```python
from build123d import *

# Parameters (mm, degrees)
SKETCH3_W            = 19.970710678
SKETCH3_H            = 7.220710678
BOSS_EXTRUDE2_DEPTH  = 10
SKETCH4_W            = 54.526496071
SKETCH4_H            = 10
BOSS_EXTRUDE3_DEPTH  = 10
SKETCH5_W            = 7.25
SKETCH5_H            = 10.1
BOSS_EXTRUDE4_DEPTH  = 20
SKETCH6_W            = 54.470710678
SKETCH6_H            = 10
BOSS_EXTRUDE5_DEPTH  = 10
SKETCH7_R            = 3
SKETCH7_R_2          = 2.998828916
CUT_EXTRUDE1_DEPTH   = 12
SKETCH8_R            = 3
CUT_EXTRUDE2_DEPTH   = 12
SKETCH9_W            = 40
SKETCH9_H            = 54.526496071
SKETCH9_W_2          = 19.9
SKETCH9_H_2          = 40
BOSS_EXTRUDE8_DEPTH  = 12
SKETCH10_W           = 20.059980773
SKETCH10_H           = 17
CUT_EXTRUDE6_DEPTH   = 8
SKETCH11_W           = 40
SKETCH11_H           = 22
BOSS_EXTRUDE9_DEPTH  = 5
SKETCH12_W           = 7.25
SKETCH12_H           = 0.1
CUT_EXTRUDE7_DEPTH   = 20
SKETCH13_W           = 20
SKETCH13_H           = 17
CUT_EXTRUDE8_DEPTH   = 20
SKETCH16_W           = 40
SKETCH16_H           = 59.526496071
BOSS_EXTRUDE11_DEPTH = 8
SKETCH17_W           = 20
SKETCH17_H           = 40
CUT_EXTRUDE10_DEPTH  = 5
SKETCH19_W           = 40
SKETCH19_H           = 30
BOSS_EXTRUDE12_DEPTH = 10
CUT_EXTRUDE11_DEPTH  = 8
SKETCH21_R           = 1.5
CUT_EXTRUDE12_DEPTH  = 30
FILLET2_R            = 4


with BuildPart() as part:
    # Sketch3 → Boss-Extrude2 (new body)
    with BuildSketch(Plane.XZ.offset(-27.7)):
        with Locations((0.014644661, 3.610355339)):
            Rectangle(SKETCH3_W, SKETCH3_H)
    extrude(amount=BOSS_EXTRUDE2_DEPTH)

    # Sketch4 → Boss-Extrude3 (add)
    with BuildSketch(Plane(origin=(10, 0, 0), x_dir=(0, 0, -1), z_dir=(1, 0, 0))):
        with Locations((20.042537357, 22.7)):
            Rectangle(SKETCH4_W, SKETCH4_H)
    extrude(amount=BOSS_EXTRUDE3_DEPTH)

    # Sketch5 → Boss-Extrude4 (add)
    with BuildSketch(Plane.ZY.offset(-10)):
        with Locations((-43.625, 22.75)):
            Rectangle(SKETCH5_W, SKETCH5_H)
    extrude(amount=BOSS_EXTRUDE4_DEPTH)

    # Sketch6 → Boss-Extrude5 (add)
    with BuildSketch(Plane.ZY.offset(10)):
        with Locations((-20.014644661, 22.7)):
            Rectangle(SKETCH6_W, SKETCH6_H)
    extrude(amount=BOSS_EXTRUDE5_DEPTH)

    # Sketch7 → Cut-Extrude1 (cut)
    with BuildSketch(Plane(origin=(0, 27.8, 0), x_dir=(1, 0, 0), z_dir=(0, 1, 0))):
        with Locations((-5.000552171, 44.609234731)):
            Circle(SKETCH7_R)
        with Locations((5.037134364, 44.609234731)):
            Circle(SKETCH7_R_2)
    extrude(amount=-CUT_EXTRUDE1_DEPTH, mode=Mode.SUBTRACT)

    # Sketch8 → Cut-Extrude2 (cut)
    with BuildSketch(Plane(origin=(0, 27.7, 0), x_dir=(1, 0, 0), z_dir=(0, 1, 0))):
        with Locations((-5, -4.75)):
            Circle(SKETCH8_R)
        with Locations((5.014644661, -4.75)):
            Circle(SKETCH8_R)
    extrude(amount=-CUT_EXTRUDE2_DEPTH, mode=Mode.SUBTRACT)

    # Sketch9 → Boss-Extrude8 (add)
    with BuildSketch(Plane.XZ.offset(-17.7)):
        with Locations((0, -20.042537357)):
            Rectangle(SKETCH9_W, SKETCH9_H)
        with Locations((0.05, -20)):
            Rectangle(SKETCH9_W_2, SKETCH9_H_2, mode=Mode.SUBTRACT)
    extrude(amount=BOSS_EXTRUDE8_DEPTH)

    # Sketch10 → Cut-Extrude6 (cut)
    with BuildSketch(Plane(origin=(0, 0, -47.305785393), x_dir=(-1, 0, 0), z_dir=(0, 0, -1))):
        with Locations((0.029990387, 14.2)):
            Rectangle(SKETCH10_W, SKETCH10_H)
    extrude(amount=-CUT_EXTRUDE6_DEPTH, mode=Mode.SUBTRACT)

    # Sketch11 → Boss-Extrude9 (add)
    with BuildSketch(Plane.XY.offset(7.220710678)):
        with Locations((0, 16.7)):
            Rectangle(SKETCH11_W, SKETCH11_H)
    extrude(amount=BOSS_EXTRUDE9_DEPTH)

    # Sketch12 → Cut-Extrude7 (cut)
    with BuildSketch(Plane(origin=(10, 0, 0), x_dir=(0, 0, -1), z_dir=(1, 0, 0))):
        with Locations((43.625, 27.75)):
            Rectangle(SKETCH12_W, SKETCH12_H)
    extrude(amount=-CUT_EXTRUDE7_DEPTH, mode=Mode.SUBTRACT)

    # Sketch13 → Cut-Extrude8 (cut)
    with BuildSketch(Plane.XY.offset(12.220710678)):
        with Locations((0, 14.2)):
            Rectangle(SKETCH13_W, SKETCH13_H)
    extrude(amount=-CUT_EXTRUDE8_DEPTH, mode=Mode.SUBTRACT)

    # Sketch16 → Boss-Extrude11 (add)
    with BuildSketch(Plane.XZ.offset(-5.7)):
        with Locations((0, -17.542537357)):
            Rectangle(SKETCH16_W, SKETCH16_H)
    extrude(amount=BOSS_EXTRUDE11_DEPTH)

    # Sketch17 → Cut-Extrude10 (cut)
    with BuildSketch(Plane(origin=(0, 5.7, 0), x_dir=(1, 0, 0), z_dir=(0, 1, 0))):
        with Locations((0, 20)):
            Rectangle(SKETCH17_W, SKETCH17_H)
    extrude(amount=-CUT_EXTRUDE10_DEPTH, mode=Mode.SUBTRACT)

    # Sketch19 → Boss-Extrude12 (add)
    with BuildSketch(Plane.XY.offset(12.220710678)):
        with Locations((0, 12.7)):
            Rectangle(SKETCH19_W, SKETCH19_H)
    extrude(amount=BOSS_EXTRUDE12_DEPTH)

    # Sketch20 → Cut-Extrude11 (cut)
    with BuildSketch(Plane.XY.offset(22.220710678)):
        with BuildLine():
            Line((-2.5, 6.2), (-2.5, 8.369872981))
            ThreePointArc((-2.5, 8.369872981), (-5, 12.7), (-2.5, 17.030127019))
            Line((-2.5, 17.030127019), (-2.5, 19.2))
            ThreePointArc((-2.5, 19.2), (0, 21.7), (2.5, 19.2))
            Line((2.5, 19.2), (2.5, 17.030127019))
            ThreePointArc((2.5, 17.030127019), (5, 12.7), (2.5, 8.369872981))
            Line((2.5, 8.369872981), (2.5, 6.2))
            ThreePointArc((2.5, 6.2), (0, 3.7), (-2.5, 6.2))
        make_face()
    extrude(amount=-CUT_EXTRUDE11_DEPTH, mode=Mode.SUBTRACT)

    # Sketch21 → Cut-Extrude12 (cut)
    with BuildSketch(Plane(origin=(0, 27.7, 0), x_dir=(1, 0, 0), z_dir=(0, 1, 0))):
        with Locations(Location((0, -15.870882648, 0), (0, 0, 270))):
            Circle(SKETCH21_R)
    extrude(amount=-CUT_EXTRUDE12_DEPTH, mode=Mode.SUBTRACT)

    # Fillet2
    # the kernel refuses this fillet: 4 mm, written as the material it takes off along each edge
    with BuildSketch(Plane(origin=(16, 23.7, 18.220710678), x_dir=(1, 0, 0), z_dir=(0, 1, 0))) as fillet2_piece_1_section:
        Polygon((0, 0), (FILLET2_R, 0), (FILLET2_R, -FILLET2_R), (0, -FILLET2_R), align=None)
    fillet2_piece_1 = extrude(amount=FILLET2_R, mode=Mode.PRIVATE)
    fillet2_piece_1 = fillet2_piece_1 - Plane(origin=(16, 23.7, 18.220710678), x_dir=(-0.7071067811865475, 0, -0.7071067811865475), z_dir=(0, 1, 0)) * Sphere(FILLET2_R, mode=Mode.PRIVATE)
    add(fillet2_piece_1, mode=Mode.SUBTRACT)
    with BuildSketch(Plane(origin=(-16, 23.7, 18.220710678), x_dir=(0, 1, 0), z_dir=(-1, 0, 0))) as fillet2_piece_2_section:
        Polygon((0, 0), (FILLET2_R, 0), (FILLET2_R, -FILLET2_R), (0, -FILLET2_R), align=None)
    fillet2_piece_2 = extrude(amount=FILLET2_R, mode=Mode.PRIVATE)
    fillet2_piece_2 = fillet2_piece_2 - Plane(origin=(-16, 23.7, 18.220710678), x_dir=(0, -0.7071067811865475, -0.7071067811865475), z_dir=(-1, 0, 0)) * Sphere(FILLET2_R, mode=Mode.PRIVATE)
    add(fillet2_piece_2, mode=Mode.SUBTRACT)
    with BuildSketch(Plane(origin=(-16, 1.7, -43.305785393), x_dir=(0, 0, -1), z_dir=(-1, 0, 0))) as fillet2_piece_3_section:
        Polygon((0, 0), (FILLET2_R, 0), (FILLET2_R, FILLET2_R), (0, FILLET2_R), align=None)
    fillet2_piece_3 = extrude(amount=FILLET2_R, mode=Mode.PRIVATE)
    fillet2_piece_3 = fillet2_piece_3 - Plane(origin=(-16, 1.7, -43.305785393), x_dir=(0, 0.7071067811865475, 0.7071067811865475), z_dir=(-1, 0, 0)) * Sphere(FILLET2_R, mode=Mode.PRIVATE)
    add(fillet2_piece_3, mode=Mode.SUBTRACT)
    with BuildSketch(Plane(origin=(-16, 1.7, 18.220710678), x_dir=(0, 0, 1), z_dir=(-1, 0, 0))) as fillet2_piece_4_section:
        Polygon((0, 0), (FILLET2_R, 0), (FILLET2_R, -FILLET2_R), (0, -FILLET2_R), align=None)
    fillet2_piece_4 = extrude(amount=FILLET2_R, mode=Mode.PRIVATE)
    fillet2_piece_4 = fillet2_piece_4 - Plane(origin=(-16, 1.7, 18.220710678), x_dir=(0, 0.7071067811865475, -0.7071067811865475), z_dir=(-1, 0, 0)) * Sphere(FILLET2_R, mode=Mode.PRIVATE)
    add(fillet2_piece_4, mode=Mode.SUBTRACT)
    with BuildSketch(Plane(origin=(16, 1.7, 18.220710678), x_dir=(1, 0, 0), z_dir=(0, -1, 0))) as fillet2_piece_5_section:
        Polygon((0, 0), (FILLET2_R, 0), (FILLET2_R, FILLET2_R), (0, FILLET2_R), align=None)
    fillet2_piece_5 = extrude(amount=FILLET2_R, mode=Mode.PRIVATE)
    fillet2_piece_5 = fillet2_piece_5 - Plane(origin=(16, 1.7, 18.220710678), x_dir=(-0.7071067811865475, 0, -0.7071067811865475), z_dir=(0, -1, 0)) * Sphere(FILLET2_R, mode=Mode.PRIVATE)
    add(fillet2_piece_5, mode=Mode.SUBTRACT)
    with BuildSketch(Plane(origin=(16, 1.7, -43.305785393), x_dir=(0, 0, -1), z_dir=(0, -1, 0))) as fillet2_piece_6_section:
        Polygon((0, 0), (FILLET2_R, 0), (FILLET2_R, FILLET2_R), (0, FILLET2_R), align=None)
    fillet2_piece_6 = extrude(amount=FILLET2_R, mode=Mode.PRIVATE)
    fillet2_piece_6 = fillet2_piece_6 - Plane(origin=(16, 1.7, -43.305785393), x_dir=(-0.7071067811865475, 0, 0.7071067811865475), z_dir=(0, -1, 0)) * Sphere(FILLET2_R, mode=Mode.PRIVATE)
    add(fillet2_piece_6, mode=Mode.SUBTRACT)
    with BuildSketch(Plane(origin=(20, 27.7, 18.220710678), x_dir=(-1, 0, 0), z_dir=(0, 0, -1))) as fillet2_piece_7:
        with BuildLine():
            CenterArc((FILLET2_R, -FILLET2_R), FILLET2_R, 90, 90)
            Line((0, -FILLET2_R), (0, 0))
            Line((0, 0), (FILLET2_R, 0))
        make_face()
    extrude(amount=75.526496071, mode=Mode.SUBTRACT)
    with BuildSketch(Plane(origin=(-20, 27.7, -57.25), x_dir=(1, 0, 0), z_dir=(0, 0, 1))) as fillet2_piece_8:
        with BuildLine():
            CenterArc((FILLET2_R, -FILLET2_R), FILLET2_R, 90, 90)
            Line((0, -FILLET2_R), (0, 0))
            Line((0, 0), (FILLET2_R, 0))
        make_face()
    extrude(amount=75.470710678, mode=Mode.SUBTRACT)
    with BuildSketch(Plane(origin=(-20, -2.3, -43.305785393), x_dir=(0, 1, 0), z_dir=(0, 0, 1)), Plane(origin=(20, -2.3, 18.220710678), x_dir=(0, 1, 0), z_dir=(0, 0, -1))) as fillet2_piece_9:
        with BuildLine():
            CenterArc((FILLET2_R, -FILLET2_R), FILLET2_R, 90, 90)
            Line((0, -FILLET2_R), (0, 0))
            Line((0, 0), (FILLET2_R, 0))
        make_face()
    extrude(amount=61.526496071, mode=Mode.SUBTRACT)
    with BuildSketch(Plane(origin=(16, -2.3, -47.305785393), x_dir=(0, 1, 0), z_dir=(-1, 0, 0)), Plane(origin=(-16, 27.7, 22.220710678), x_dir=(0, 0, -1), z_dir=(1, 0, 0))) as fillet2_piece_10:
        with BuildLine():
            CenterArc((FILLET2_R, -FILLET2_R), FILLET2_R, 90, 90)
            Line((0, -FILLET2_R), (0, 0))
            Line((0, 0), (FILLET2_R, 0))
        make_face()
    extrude(amount=32, mode=Mode.SUBTRACT)
    with BuildSketch(Plane(origin=(16, -2.3, 22.220710678), x_dir=(0, 1, 0), z_dir=(-1, 0, 0))) as fillet2_piece_11:
        with BuildLine():
            CenterArc((FILLET2_R, FILLET2_R), FILLET2_R, 180, 90)
            Line((0, FILLET2_R), (0, 0))
            Line((0, 0), (FILLET2_R, 0))
        make_face()
    extrude(amount=32, mode=Mode.SUBTRACT)
    with BuildSketch(Plane(origin=(-20, 1.7, -47.305785393), x_dir=(1, 0, 0), z_dir=(0, 1, 0))) as fillet2_piece_12:
        with BuildLine():
            CenterArc((FILLET2_R, -FILLET2_R), FILLET2_R, 90, 90)
            Line((0, -FILLET2_R), (0, 0))
            Line((0, 0), (FILLET2_R, 0))
        make_face()
    extrude(amount=26, mode=Mode.SUBTRACT)
    with BuildSketch(Plane(origin=(20, 37.7, -47.305785393), x_dir=(-1, 0, 0), z_dir=(0, -1, 0))) as fillet2_piece_13:
        with BuildLine():
            CenterArc((FILLET2_R, -FILLET2_R), FILLET2_R, 90, 90)
            Line((0, -FILLET2_R), (0, 0))
            Line((0, 0), (FILLET2_R, 0))
        make_face()
    extrude(amount=36, mode=Mode.SUBTRACT)
    with BuildSketch(Plane(origin=(20, 23.7, 22.220710678), x_dir=(0, 0, -1), z_dir=(0, -1, 0))) as fillet2_piece_14:
        with BuildLine():
            CenterArc((FILLET2_R, -FILLET2_R), FILLET2_R, 90, 90)
            Line((0, -FILLET2_R), (0, 0))
            Line((0, 0), (FILLET2_R, 0))
        make_face()
    extrude(amount=22, mode=Mode.SUBTRACT)
    with BuildSketch(Plane(origin=(-20, 1.7, 22.220710678), x_dir=(1, 0, 0), z_dir=(0, 1, 0))) as fillet2_piece_15:
        with BuildLine():
            CenterArc((FILLET2_R, FILLET2_R), FILLET2_R, 180, 90)
            Line((0, FILLET2_R), (0, 0))
            Line((0, 0), (FILLET2_R, 0))
        make_face()
    extrude(amount=22, mode=Mode.SUBTRACT)


solid = part.part
```
The listing builds one solid part. Answer for the finished solid, in the listing's coordinates (mm). A direction names the side the tool comes from. Give positions to 0.01 mm unless a question says otherwise; leave off trailing zeros. Order: outer loops, then holes, each group sorted by start corner. A loop starts at its lowest first (then second) coordinate and runs counter-clockwise, first axis right, second up.
1) Find section A-A on x = 0. Give the number of separate pieces and of enclosed holes in the cut face, then the cut area to 3 significant figures.
Reported:
separate pieces: 4
enclosed holes: 0
area: 483 mm2
2) Find section C-C on z = -32.5. Write down the section's boundary in (x, y).
Reported:
outline: (-20, 1.7) arc R4 ccw to (-16, -2.3) - (16, -2.3) arc R4 ccw to (20, 1.7) - (20, 23.7) arc R4 ccw to (16, 27.7) - (10, 27.7) - (10, 0.7) - (-10, 0.7) - (-10, 5.7) - (-9.9, 5.7) - (-9.9, 17.7) - (-10, 17.7) - (-10, 27.7) - (-16, 27.7) arc R4 ccw to (-20, 23.7) - close
3) Determine the mould class of faces 1 (the face through (18.797, 26.559, -14.084)), 2 (the face through (0, 0.7, -20)), 3 (the face through (0.22, -1.16, 21.02)) for opening direction X: pulls with the +X half, pulls with the -X half, needs draft (parallel to the pull), parting line crosses it, or undercut.
Reported:
face 1: pulls with the +X half
face 2: undercut
face 3: needs draft
4) Consider line 1 along Z through (x, y) = (0, 23); line 2 along Z through (x, y) = (-5, 24); line 3 along Z through (x, y) = (6, 2). Determine where each line is inside the solid, lowest interval first.
Reported:
line 1: z = -47.25 to -40, 0 to 14.37, 17.37 to 22.22
line 2: z = -41.61 to -40, 0 to 1.75, 7.22 to 22.21
line 3: z = -47.31 to -40, 0 to 22.22
5) Find section D-D on y = 10.5. Write down the section's boundary in (x, z).
Reported:
outline: (-20, -43.31) arc R4 ccw to (-16, -47.31) - (-10.06, -47.31) - (-10.06, -39.31) - (-9.9, -39.31) - (-9.9, -7.78) - (-10, -7.78) - (-10, 12.22) - (10, 12.22) - (10, -47.31) - (16, -47.31) arc R4 ccw to (20, -43.31) - (20, 18.22) arc R4 ccw to (16, 22.22) - (4.49, 22.22) - (4.49, 14.22) - (-4.49, 14.22) - (-4.49, 22.22) - (-16, 22.22) arc R4 ccw to (-20, 18.22) - close
6) Find section B-B on z = 4.75. Write down the section's boundary in (x, y).
Reported:
outline: (-20, 1.7) arc R4 ccw to (-16, -2.3) - (16, -2.3) arc R4 ccw to (20, 1.7) - (20, 23.7) arc R4 ccw to (16, 27.7) - (8.01, 27.7) - (8.01, 22.7) - (10, 22.7) - (10, 5.7) - (-10, 5.7) - (-10, 27.7) - (-16, 27.7) arc R4 ccw to (-20, 23.7) - close; (-9.97, 22.7) - (-8, 22.7) - (-8, 27.7) - (-9.97, 27.7) - close; (-2, 22.7) - (2.01, 22.7) - (2.01, 27.7) - (-2, 27.7) - close
7) For faces 4 (the face through (-13, 23, -47.25)), 5 (the face through (0, 22.7, -43)), 6 (the face through (2.5, 7, 18)), 7 (the face through (0.224, -1.097, -46.165)), 8 (the face through (-5, 25, 7.221)), determine the directions among +Z, -Z, +X, -X, +Y, -Y from which every point of the face is accessible in a straight line to the end or side of a thin tool.
Reported:
face 4: -Z, -X, +Y
face 5: -Z
face 6: +Z
face 7: -Z, +X, -X, -Y
face 8: +Y
8) Given P1, Ø3, axis at x = -9, y = 20.5, coming from the -Z side; P2, Ø3, axis at x = 6, z = -7, coming from the +Y side, each flat-ended and moving along its own axis, determine where each tip first touches the part or whether it passes through.
Reported:
P1: stops at z = -47.25
P2: stops at y = 0.7
